Can you work these out from the drawing? Everything is in mm from the part's minimum corner. A direction names the side the tool comes from. Give positions to 0.01 mm unless a question says otherwise; leave off trailing zeros. Loops run counter-clockwise (first coordinate to the right, second up) from the corner with the lowest first, then second, coordinate; pieces in that order, holes last. Notation, with made-up numbers: (60.5, 11.25) -> (105.5, 11.25) arc R23 ccw to (105.5, 36.25) -> close; hole circle Ø11 at (9, 64). An arc over 180 degrees is marked (long way). Return JSON: item names as keys, results as strings. Group by question number.
Q1. Suppose I cut it at B-B, the plane z = 28. Please give me the cut outline in (x, y) (3 decimals).
Q2. Suppose I cut it at C-C, the plane x = 46.5. Please give me the cut outline in (y, z).
Q3. Will these pins go through, and if not, where does the flat tip stop? pin 1 (13.5 mm diameter, centred on x = 34.5, z = 28.5, fed in from +Y); pin 2 (10 mm diameter, centred on y = 27, z = 38, fed in from -X) (3 decimals); pin 3 (13.5 mm diameter, centred on y = 25.5, z = 19.5, fed in from +X) (3 decimals).
Q4. Suppose I cut it at D-D, the plane y = 10.5. Please give me the cut outline in (x, z) (3 decimals), and give its area (3 significant figures).
Q5. Suppose I cut it at A-A, the plane y = 102. Please give me the cut outline in (x, z), and give its area (3 significant figures).
Q6. I need wall thicknesses on line 1 along Z through (x, y) = (5.5, 76); line 2 along X through (y, z) = (5, 28) (3 decimals); line 3 along Y through (x, z) = (19, 26.5). Which ranges of each line are inside material? Lowest first, please. Write a range as [from, to].
Q7. Thinking about a two-plate mould opening in X: for the marked faces 1, 2, 3 and 4, which applies, pulls with the +X half, pulls with the -X half, needs draft (parallel to the pull), parting line crosses it, or undercut?
Q8. Which directions (+Z, -Z, +X, -X, +Y, -Y) give clear straight access to the entire face, cutting with the end or side of a thin tool? Please do the marked faces 5 and 6.
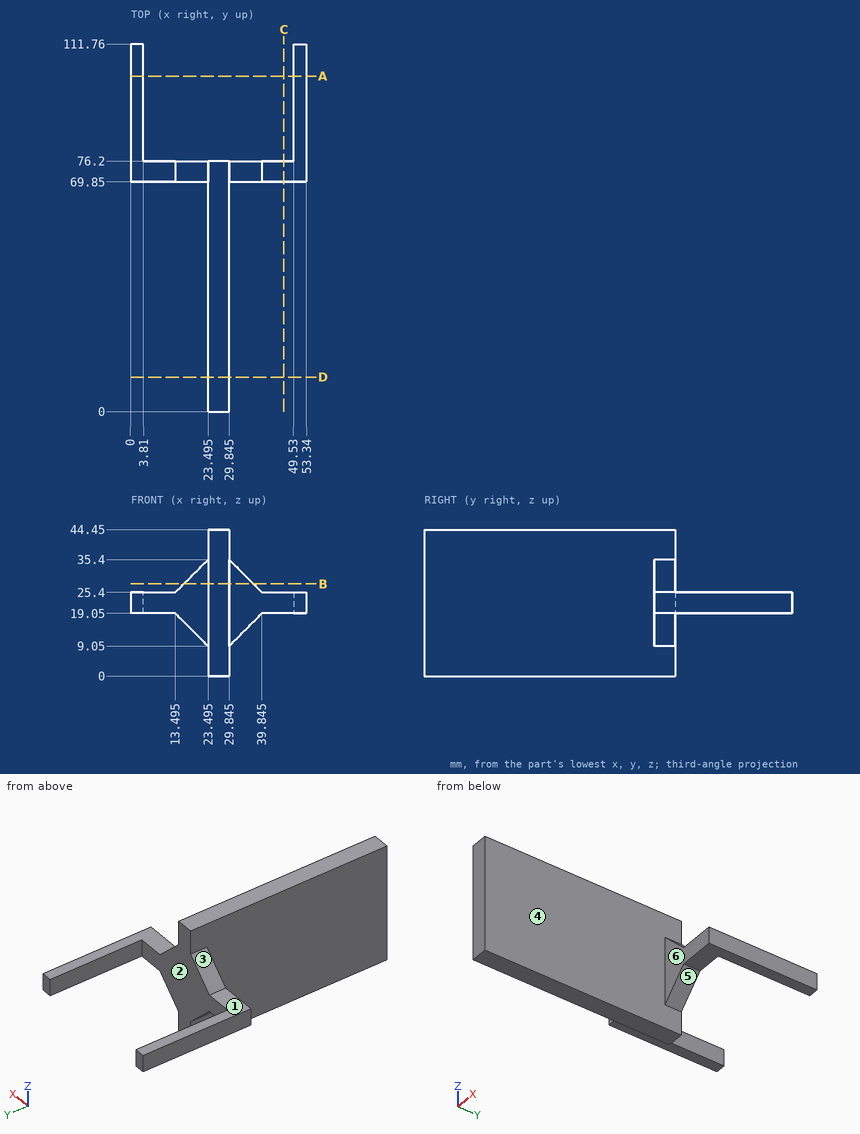
Ans:
{
 "1": {"outline": "(16.095, 69.85) -> (23.495, 69.85) -> (23.495, 0) -> (29.845, 0) -> (29.845, 69.85) -> (37.245, 69.85) -> (37.245, 76.2) -> (16.095, 76.2) -> close"},
 "2": {"outline": "(69.85, 19.05) -> (76.2, 19.05) -> (76.2, 25.4) -> (69.85, 25.4) -> close"},
 "3": {"pin 1": "stops at y = 76.2", "pin 2": "stops at x = 23.495", "pin 3": "stops at x = 29.845"},
 "4": {"outline": "(23.495, 0) -> (29.845, 0) -> (29.845, 44.45) -> (23.495, 44.45) -> close", "area": "282 mm^2"},
 "5": {"outline": "(0, 19.05) -> (3.81, 19.05) -> (3.81, 25.4) -> (0, 25.4) -> close; (49.53, 19.05) -> (53.34, 19.05) -> (53.34, 25.4) -> (49.53, 25.4) -> close", "area": "48.4 mm^2"},
 "6": {"line 1": "z = [19.05, 25.4]", "line 2": "x = [23.495, 29.845]", "line 3": "y = [69.85, 76.2]"},
 "7": {"face 1": "needs draft", "face 2": "undercut", "face 3": "pulls with the -X half", "face 4": "pulls with the +X half"},
 "8": {"face 5": "-Z, +X, +Y, -Y", "face 6": "+Z, -Z, +X, -Y"}
}
